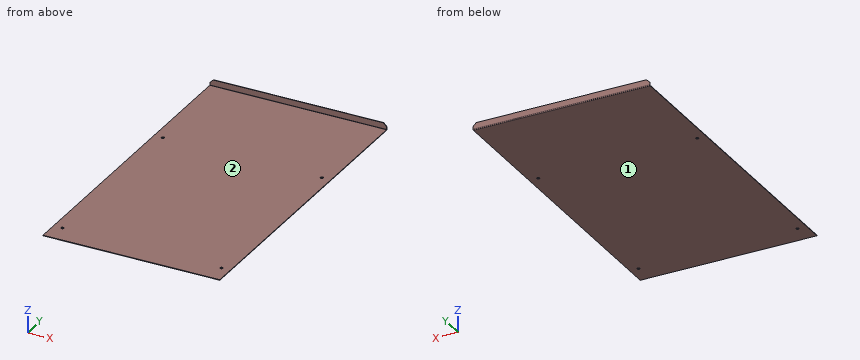
from build123d import *

# Parameters (mm, degrees)
SKETCH1_W           = 266.4508474
SKETCH1_H           = 475
BASE_FLANGE1_DEPTH  = 0.889
SKETCH6_R           = 2.25
CUT_EXTRUDE1_DEPTH  = 0.889
EDGE_FLANGE3_DEPTH  = 266.4508474
BREAK_CORNER1_START = 0.381
BREAK_CORNER1_DEPTH = 0.889


# Read off the part's stored shape, not the designer's step: Break-Corner1
# Sheet-metal steps are written as plain solids
with BuildPart() as part:
    # Sketch1 → Base-Flange1 (new body)
    with BuildSketch(Plane.XY):
        with Locations((0, -237.5)):
            Rectangle(SKETCH1_W, SKETCH1_H)
    extrude(amount=-BASE_FLANGE1_DEPTH)

    # Sketch6 → Cut-Extrude1 (cut)
    with BuildSketch(Plane(origin=(0, 0, -0.889), x_dir=(-1, 0, 0), z_dir=(0, 0, -1))):
        with Locations((-119.8215307, -158.867160024)):
            Circle(SKETCH6_R)
        with Locations((119.8215307, -158.867160024)):
            Circle(SKETCH6_R)
        with Locations((-119.8215307, -445)):
            Circle(SKETCH6_R)
        with Locations((119.8215307, -445)):
            Circle(SKETCH6_R)
    extrude(amount=-CUT_EXTRUDE1_DEPTH, mode=Mode.SUBTRACT)

    # Edge-Flange3 section (across the edge) → Edge-Flange3 (add)
    with BuildSketch(Plane(origin=(133.2254237, 0.381, 0), x_dir=(0, -1, 0), z_dir=(-1, 0, 0))):
        with BuildLine():
            Line((-0.889, 0.381), (-0.889, 9.111))
            Line((-0.889, 9.111), (0, 9.111))
            Line((0, 9.111), (0, 0.381))
            ThreePointArc((0, 0.381), (0.111592316, 0.111592316), (0.381, 0))
            Line((0.381, 0), (0.381, -0.889))
            ThreePointArc((0.381, -0.889), (-0.517025612, -0.517025612), (-0.889, 0.381))
        make_face()
    extrude(amount=EDGE_FLANGE3_DEPTH)

    # Break-Corner1 outline → Break-Corner1 (cut)
    with BuildSketch(Plane(origin=(0, 0, 0), x_dir=(1, 0, 0), z_dir=(0, 1, 0)).offset(BREAK_CORNER1_START)):
        Polygon((-133.2254237, -9.111), (-128.2254237, -9.111), (-133.2254237, -4.111), align=None)
        Polygon((133.2254237, -4.111), (128.2254237, -9.111), (133.2254237, -9.111), align=None)
    extrude(amount=BREAK_CORNER1_DEPTH, mode=Mode.SUBTRACT)


solid = part.part
Can you work these out from the model? Positions are in its coordinate system, mm. Face numbers are marked on the shaded views. A direction names the side the tool comes from. Give positions to 0.01 mm unless a question says otherwise; leave off trailing zeros. Write each loop counter-clockwise with the first axis right and the second up, starting at its lowest first coordinate (ties: lowest second). Pieces come first, ordered by that corner, then holes. Notation, with made-up numbers: (42.25, 36.5) -> (51.25, 36.5) arc R11 ccw to (51.25, 51.5) -> close; hole circle Ø6 at (-12, 59). An arc over 180 degrees is marked (long way). Answer as a JSON object with one key per item and string values. Group by question number.
Item 1: Suppose I cut it at B-B (y = -91). Please give me the cut outline in (x, z).
Item 2: I'm going to push flat-ended pins straight in: P1, Ø6, axis at x = -119.82, y = -445, coming from the +Z side; P2, Ø1.5, axis at y = -109.5, z = 0.5, coming from the -X side; P3, Ø2.5, axis at x = -49, z = 7, coming from the -Y side. Where does each tip first touch, or does it pass through?
Item 3: Suppose I cut it at A-A (x = -92.5). Please give me the cut outline in (y, z).
Item 4: Please list where these lines run through material, in increasing order: line 1 (X direction, y = -445, z = -0.4); line 2 (Z direction, x = -6, y = -380.5); line 3 (Y direction, x = -94, z = 7.75). Write a range as [from, to].
Item 5: Suppose I cut it at C-C (z = 6). Please give me the cut outline in (x, y), plus the area to 3 significant figures.
Item 6: For the marked faces 1 and 2, which set-ups out of +Z, -Z, +X, -X, +Y, -Y let a thin tool reach every point of the face, with its end or its side?
Findings:
{
 "1": {"outline": "(-133.23, -0.89) -> (133.23, -0.89) -> (133.23, 0) -> (-133.23, 0) -> close"},
 "2": {"P1": "stops at z = 0", "P2": "stops at x = -133.23", "P3": "stops at y = 0.38"},
 "3": {"outline": "(-475, -0.89) -> (0, -0.89) arc R1.27 ccw to (1.27, 0.38) -> (1.27, 9.11) -> (0.38, 9.11) -> (0.38, 0.38) arc R0.38 cw to (0, 0) -> (-475, 0) -> close"},
 "4": {"line 1": "x = [-133.23, -122.07], [-117.57, 117.57], [122.07, 133.23]", "line 2": "z = [-0.89, 0]", "line 3": "y = [0.38, 1.27]"},
 "5": {"outline": "(-131.34, 0.38) -> (131.34, 0.38) -> (131.34, 1.27) -> (-131.34, 1.27) -> close", "area": "234 mm²"},
 "6": {"face 1": "-Z, +X, -X, +Y, -Y", "face 2": "+Z, +X, -X, -Y"}
}
